from build123d import *

# Parameters (mm, degrees)
SKETCH1_R           = 113.336684476
BOSS_EXTRUDE1_DEPTH = 2
SKETCH3_R           = 113.336684476
BOSS_EXTRUDE2_DEPTH = 33
BOSS_EXTRUDE2_DRAFT = -66
SKETCH4_R           = 187.455898015
BOSS_EXTRUDE3_DEPTH = 5
SKETCH6_W           = 105.518937327
SKETCH6_H           = 48.279891136
SKETCH7_R           = 25
CUT_EXTRUDE1_DEPTH  = 30.552152957


with BuildPart() as part:
    # Sketch1 → Boss-Extrude1 (new body)
    with BuildSketch(Plane.XY):
        with Locations((-74.414862174, -31.38339944)):
            Circle(SKETCH1_R)
    extrude(amount=BOSS_EXTRUDE1_DEPTH)


with BuildPart() as boss_extrude2_tool:
    # Sketch3 → Boss-Extrude2 (with draft: the straight prism first)
    with BuildSketch(Plane.XY.offset(2)):
        with Locations((-74.414862174, -31.38339944)):
            Circle(SKETCH3_R)
    extrude(amount=BOSS_EXTRUDE2_DEPTH)
    # Boss-Extrude2: the draft: its side faces are tilted about the plane it starts from
    boss_extrude2_sides = [boss_extrude2_tool.faces().sort_by_distance(p)[0] for p in [
        (-187.75154665, -31.38339944, 18.5),
    ]]
    draft(boss_extrude2_sides, Plane.XY.offset(2), BOSS_EXTRUDE2_DRAFT)


with BuildPart() as part_1:
    add(part.part)

    # Boss-Extrude2: add boss_extrude2_tool
    add(boss_extrude2_tool.part)

    # Sketch4 → Boss-Extrude3 (add)
    with BuildSketch(Plane.XY.offset(35)):
        with Locations((-74.414862174, -31.38339944)):
            Circle(SKETCH4_R)
    extrude(amount=BOSS_EXTRUDE3_DEPTH)

    # Sketch6 → Cut-Revolve1 (revolve, cut)
    with BuildSketch(Plane(origin=(0, -31.38339944, 0), x_dir=(-1, 0, 0), z_dir=(0, -1, 0))):
        with Locations((21.655393511, -32.895152959)):
            Rectangle(SKETCH6_W, SKETCH6_H)
    revolve(axis=Axis((-74.414862174, -31.38339944, -21.108642796), (0, 0, -1)), mode=Mode.SUBTRACT)

    # Sketch7 → Cut-Extrude1 (cut)
    with BuildSketch(Plane(origin=(0, 0, 0), x_dir=(-1, 0, 0), z_dir=(0, 0, -1))):
        with Locations((-74.30011683, -31.38339944)):
            Circle(SKETCH7_R)
        with Locations((74.414862174, -180.098378444)):
            Circle(SKETCH7_R)
        with Locations((74.414862174, 117.331579563)):
            Circle(SKETCH7_R)
        with Locations((223.129841177, -31.38339944)):
            Circle(SKETCH7_R)
    extrude(amount=-CUT_EXTRUDE1_DEPTH, mode=Mode.SUBTRACT)


solid = part_1.part
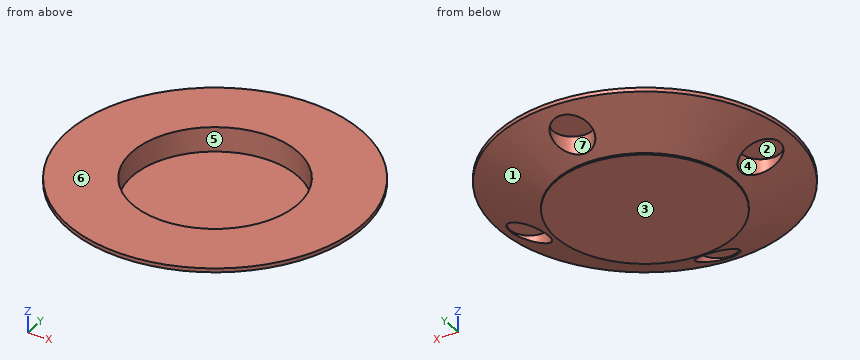
The listing builds one solid part. Answer for the finished solid, in the listing's coordinates (mm). Face numbers are marked on the shaded views. A direction names the side the tool comes from. Coordinates: 2 decimals unless noted, no trailing zeros.
Q1. Consider line 1 (X direction, y = -61, z = 13); line 2 (X direction, y = -41, z = 27); line 3 (Z direction, x = -86, y = -39). Determine where each line is inside the solid, lowest interval first.
Q2. For a pull along X with two mould halves and no side action, classify the marked faces 1, 2, 3 and 4 as pulls with the +X half, pulls with the -X half, needs draft (parallel to the pull), parting line crosses it, or undercut.
Q3. Given P1, Ø15, axis at x = -69, y = 106.5, coming from the -Z side; P2, Ø10, axis at x = -122.5, y = -57, coming from the +Z side; P3, Ø8, axis at y = -113.5, z = 34.5, coming from the +X side, each flat-ended and moving along its own axis, determine where each tip first touches the part or whether it passes through.
Q4. Which of the six approach directions +Z, -Z, +X, -X, +Y, -Y give full straight-line access (tool end or side, diameter ignored) to the marked faces 5, 6 and 7?
Answers follow:
1. line 1: x = -209.24 to -175.69, 26.86 to 60.41
1. line 2: x = -200.05 to -179.49, 30.66 to 51.22
1. line 3: z = 0 to 8.76
2. face 1: parting line crosses it
2. face 2: undercut
2. face 3: needs draft
2. face 4: undercut
3. P1: stops at z = 30.55
3. P2: stops at z = 8.76
3. P3: stops at x = 95.97
4. face 5: +Z
4. face 6: +Z, +X, -X, +Y, -Y
4. face 7: -Z
